Here's how the part is built. I have some questions about the finished solid (model axes, mm). A direction names the side the tool comes from. Round coordinates to 2 decimals unless told otherwise and drop trailing zeros. Write each loop counter-clockwise with the first axis right and the second up, starting at its lowest first coordinate (ties: lowest second). Pieces come first, ordered by that corner, then holes. Notation, with made-up numbers: (48, 59.25) - (64, 59.25) arc R23 cw to (64, 79.25) - close; hole circle Ø6 at (18, -9.75). An arc over 180 degrees is marked (long way). Write item = value, one per line. Start each with the question number.
Item 1: If we section it at A-A (z = 17.75): Please give me the cut outline in (x, y).
Item 2: If I drill on line 1 along X through (y, z) = (4.5, 11.25); line 2 along X through (y, z) = (16.25, 18.25); line 3 along X through (y, z) = (16, 7.5), over which ranges is the centre line in solid material (lowest first)? Write a range as [from, to].
Item 3: Thinking about a two-plate mould opening in Z: for faces 3 (the face through (10, 20, 8)), 4 (the face through (15, 10, 0)), 5 (the face through (15, 10, 15)), which applies, pulls with the +Z half, pulls with the -Z half, needs draft (parallel to the pull), parting line crosses it, or undercut?
Item 4: If we section it at C-C (x = 13.75): Please give me the cut outline in (y, z).
Item 5: Which directions (+Z, -Z, +X, -X, +Y, -Y) give clear straight access to the entire face, cutting with the end or side of a thin tool? Please do faces 1 (the face through (5, 10, 15)), 2 (the face through (20, 10, 10)).
Item 6: If we section it at D-D (y = 2.75): Please give me the cut outline in (x, z).
Item 7: For P1, Ø10, axis at x = 3, y = 4, coming from the +Z side, with a flat end and sliding along its axis, tell me the tip position at first contact or that it passes through.
Item 8: If we section it at B-B (z = 11.5): Please give me the cut outline in (x, y).
```python
from build123d import *

# Parameters (mm, degrees)
SKETCH1_W           = 20
SKETCH1_H           = 20
BOSS_EXTRUDE1_DEPTH = 20
CUT_EXTRUDE1_DEPTH  = 20
CUT_EXTRUDE2_DEPTH  = 20


with BuildPart() as part:
    # Sketch1 → Boss-Extrude1 (new body)
    with BuildSketch(Plane.XY):
        with Locations((10, 10)):
            Rectangle(SKETCH1_W, SKETCH1_H)
    extrude(amount=BOSS_EXTRUDE1_DEPTH)

    # Sketch2 → Cut-Extrude1 (cut)
    with BuildSketch(Plane(origin=(0, 20, 0), x_dir=(1, 0, 0), z_dir=(0, 1, 0))):
        Polygon((0, 0), (10, 0), (0, -10), align=None)
    extrude(amount=-CUT_EXTRUDE1_DEPTH, mode=Mode.SUBTRACT)

    # Sketch3 → Cut-Extrude2 (cut)
    with BuildSketch(Plane(origin=(0, 20, 0), x_dir=(1, 0, 0), z_dir=(0, 1, 0))):
        Polygon((20, -20), (10, -10), (0, -20), align=None)
    extrude(amount=-CUT_EXTRUDE2_DEPTH, mode=Mode.SUBTRACT)


solid = part.part
```
Reply:
q1.outline = (0, 0) - (2.25, 0) - (2.25, 20) - (0, 20) - close; (17.75, 0) - (20, 0) - (20, 20) - (17.75, 20) - close
q2.line_1 = [0, 8.75], [11.25, 20]
q2.line_2 = [0, 1.75], [18.25, 20]
q2.line_3 = [2.5, 20]
q3.face_3 = needs draft
q3.face_4 = pulls with the -Z half
q3.face_5 = pulls with the +Z half
q4.outline = (0, 0) - (20, 0) - (20, 13.75) - (0, 13.75) - close
q5.face_1 = +Z, +Y, -Y
q5.face_2 = +Z, -Z, +X, +Y, -Y
q6.outline = (0, 10) - (10, 0) - (20, 0) - (20, 20) - (10, 10) - (0, 20) - close
q7.P1 = 20
q8.outline = (0, 0) - (8.5, 0) - (8.5, 20) - (0, 20) - close; (11.5, 0) - (20, 0) - (20, 20) - (11.5, 20) - close
